Autodesk Inventor part; units mm, degrees
ref_plane "Work Plane1" through (0, 7, 0) normal (0, 1, 0) x (-1, 0, 0)
ref_plane "YZ Plane" through (0, 0, 0) normal (1, 0, 0) x (0, 1, 0)
ref_plane "XY Plane" through (0, 0, 0) normal (0, 0, 1) x (1, 0, 0)
sketch "Sketch1" plane through (0, 0, 0) normal (0, 0, 1) x (1, 0, 0)
  circle A0 centre (0, 0) radius 7
  circle A1 centre (0, 0) radius 4
  dimension "d0" = 14
  dimension "d1" = 8
extrude "Extrusion1" add sketch "Sketch1" along normal blind 25.4
fillet "Fillet1" radius 1 2 edges at (-7, 0, 25.4) (-7, 0, 0)
fillet "Fillet2" radius 1 2 edges at (-4, 0, 25.4) (-4, 0, 0)
ref_plane "Work Plane1" through (0, 7, 0) normal (0, 1, 0) x (-1, 0, 0)
sketch "Sketch2" plane through (0, 7, 0) normal (0, 1, 0) x (-1, 0, 0)
  circle A0 centre (0, 5) radius 2
  circle A1 centre (0, 20.4) radius 2
  line L0 (-6, 25.4) -> (6, 25.4)
  point P0 (0, 0)
  dimension "d6" = 4
  dimension "d7" = 5
  dimension "d8" = 5
extrude "Extrusion2" cut sketch "Sketch2" against normal up to next
thread "Thread1"
thread "Thread2"
equation "\"d8\" = d7"
properties part number "AcopleMotor"
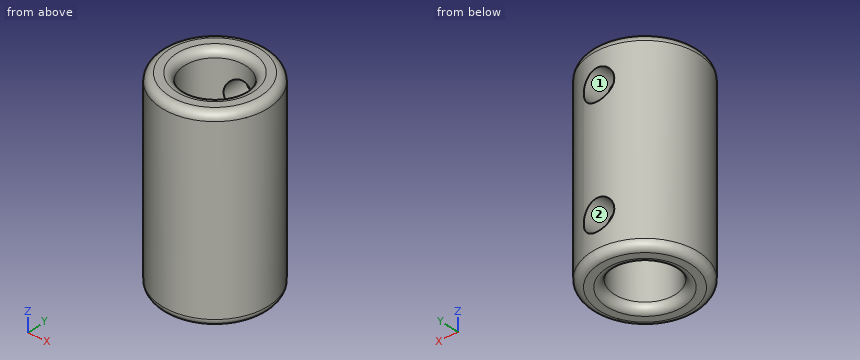
Geometry check sheet. Reference: the model listing, model coordinates, mm. Face numbers are marked on the shaded views. Round coordinates to 2 decimals unless told otherwise and drop trailing zeros. Order: outer loops, then holes, each group sorted by start corner. A loop starts at its lowest first (then second) coordinate and runs counter-clockwise, first axis right, second up. Notation, with made-up numbers: (35.5, 2) - (71.5, 2) arc R7 cw to (71.5, 11) - close; hole circle Ø4 at (23.25, 20.5). An arc over 180 degrees is marked (long way). Use a Markdown table: item, result. Add a question column.
1) Section check D-D (z = 20.4). Record the cut outline in (x, y), then the cut area to 3 significant figures.
2) Section check B-B (y = 0). Record the cut outline in (x, z).
3) Gauge pin test, flat end, axial feed: P1, Ø3, axis at y = 3, z = 17, coming from the -X side. Record the tip position at first contact, or that the pin passes through.
4) Section check A-A (x = 0). Record the cut outline in (y, z), then the cut area to 3 significant figures.
5) Thickness scan on line 1 along Z through (x, y) = (0, 5.2); line 2 along Y through (x, z) = (0, 12); line 3 along Z through (x, y) = (0, 4.6). Record the ranges inside material, lowest first.
6) Mould release check, pull along Z, two halves, no side actions. Record for the marked faces 1 and 2: released by +Z, released by -Z, zero draft, split by the parting line, or undercut.
7) Section check C-C (z = 17.5). Record the cut outline in (x, y).
Established:
| question | item | result |
|---|---|---|
| 1 | outline | (-2, 3.46) - (-2, 6.71) arc R7 ccw (long way) to (2, 6.71) - (2, 3.46) arc R4 cw (long way) to start |
| 1 | area | 91.4 mm2 |
| 2 | outline | (-7, 1) arc R1 ccw to (-6, 0) - (-5, 0) arc R1 ccw to (-4, 1) - (-4, 24.4) arc R1 ccw to (-5, 25.4) - (-6, 25.4) arc R1 ccw to (-7, 24.4) - close; (4, 1) arc R1 ccw to (5, 0) - (6, 0) arc R1 ccw to (7, 1) - (7, 24.4) arc R1 ccw to (6, 25.4) - (5, 25.4) arc R1 ccw to (4, 24.4) - close |
| 3 | P1 | x = -6.84 |
| 4 | outline | (-7, 1) arc R1 ccw to (-6, 0) - (-5, 0) arc R1 ccw to (-4, 1) - (-4, 24.4) arc R1 ccw to (-5, 25.4) - (-6, 25.4) arc R1 ccw to (-7, 24.4) - close; (4, 1) arc R1 ccw to (5, 0) - (6, 0) arc R1 ccw to (7, 1) - (7, 3) - (4, 3) - close; (4, 7) - (7, 7) - (7, 18.4) - (4, 18.4) - close; (4, 22.4) - (7, 22.4) - (7, 24.4) arc R1 ccw to (6, 25.4) - (5, 25.4) arc R1 ccw to (4, 24.4) - close |
| 4 | area | 127 mm2 |
| 5 | line 1 | 0 to 3, 7 to 18.4, 22.4 to 25.4 |
| 5 | line 2 | -7 to -4, 4 to 7 |
| 5 | line 3 | 0.08 to 3, 7 to 18.4, 22.4 to 25.32 |
| 6 | face 1 | undercut |
| 6 | face 2 | undercut |
| 7 | outline | circle Ø14 at (0, 0); hole circle Ø8 at (0, 0) |
